Work out the finished part from the listing and answer in its coordinate system (mm). A direction names the side the tool comes from. Round coordinates to 2 decimals unless told otherwise and drop trailing zeros. Loops run counter-clockwise (first coordinate to the right, second up) from the corner with the lowest first, then second, coordinate; pieces in that order, holes last.
```python
from build123d import *

# Parameters (mm, degrees)
BOSS_EXTRUDE1_DEPTH = 1


with BuildPart() as part:
    # Sketch1 → Revolve1 (revolve)
    with BuildSketch(Plane.XY):
        with BuildLine():
            Line((2.192086479, -4.705335748), (4.85, -6.209624758))
            Line((4.85, -6.209624758), (5, -6.209624758))
            Line((5, -6.209624758), (5, -7.037825562))
            Line((5, -7.037825562), (1.5, -7.037825562))
            Line((1.5, -7.037825562), (1.5, -15.067944601))
            Line((1.5, -15.067944601), (0, -15.067944601))
            Line((0, -15.067944601), (0, 4.709624758))
            ThreePointArc((0, 4.709624758), (4.570709757, 1.135419606), (2.203858582, -4.162159622))
            ThreePointArc((2.203858582, -4.162159622), (2.035645477, -4.430229616), (2.192086479, -4.705335748))
        make_face()
    revolve(axis=Axis((0, 4.709624758, 0), (0, -1, 0)))

    # Sketch3 → Boss-Extrude1 (add)
    with BuildSketch(Plane.XZ.offset(7.037825562)):
        Polygon((5.773502692, 0), (2.886751346, 5), (-2.886751346, 5), (-5.773502692, 0), (-2.886751346, -5), (2.886751346, -5), align=None)
    extrude(amount=-BOSS_EXTRUDE1_DEPTH)


solid = part.part
```
1. Which of the six approach directions +Z, -Z, +X, -X, +Y, -Y give full straight-line access (tool end or side, diameter ignored) to faces 5 (the face through (-1.5, -11.11, 0.07)), 6 (the face through (0, -15.068, 0))?
Answer key:
face 5: -Y
face 6: +Z, -Z, +X, -X, -Y
2. Find section A-A (x = 0). Write down the section's boundary in (y, z), then the cut area to 3 significant figures.
Answer key:
outline: (-15.07, -1.5) - (-7.04, -1.5) - (-7.04, -5) - (-6.04, -5) - (-6.04, -4.55) - (-4.71, -2.19) arc R0.31 cw to (-4.16, -2.2) arc R4.71 ccw (long way) to (-4.16, 2.2) arc R0.31 cw to (-4.71, 2.19) - (-6.04, 4.55) - (-6.04, 5) - (-7.04, 5) - (-7.04, 1.5) - (-15.07, 1.5) - close
area: 113 mm2
3. Given pin 1 (2 mm diameter, centred on x = -1.5, y = -8.5, fed in from -Z); pin 2 (4 mm diameter, centred on x = -4, y = 2.5, fed in from -Z); pin 3 (2 mm diameter, centred on x = 0, z = 3, fed in from -Y), each flat-ended and moving along its own axis, determine where each tip first touches the part or whether it passes through.
Answer key:
pin 1: stops at z = -1.41
pin 2: stops at z = -3.85
pin 3: stops at y = -7.04
4. Consider probe 1 along Y at (x, z) = (2, 4.5); probe 2 along Y at (x, z) = (-1.25, 3.5); probe 3 along Y at (x, z) = (-3.5, 1.5). Determine where each line is inside the solid, lowest interval first.
Answer key:
probe 1: y = -7.04 to -6.04
probe 2: y = -7.04 to -5.57, -2.89 to 2.89
probe 3: y = -7.04 to -5.62, -2.77 to 2.77
5. Find section B-B (y = -9). Write down the section's boundary in (x, z).
Answer key:
outline: circle Ø3 at (0, 0)
6. Determine the mould class of faces 1 (the face through (-2.34, -4.79, 0.1)), 2 (the face through (3, -6.038, 4)), 3 (the face through (-4.31, -6.545, 2.535)), 4 (the face through (1.2, -7.038, 1.2)) for opening direction Y: +Y half, -Y half, draft (parallel to the pull), parting line (faces both ways), or undercut.
Answer key:
face 1: undercut
face 2: undercut
face 3: draft
face 4: -Y half
